Autodesk Fusion 360 part; units mm, degrees
sketch "Sketch1" plane through (0, 0, 0) normal (0, 1, 0) x (1, 0, 0)
  arc A0 (28, 0) -> (-28, 0) centre (0, 0) ccw
  line L0 (-28, 0) -> (-28, -3)
  line L1 (0, -1.75) -> (0, -22.5)
  line L2 (28, 0) -> (28, -3)
  line L3 (-30, 0) -> (-30, -3)
  arc A1 (30, 0) -> (-30, 0) centre (0, 0) ccw
  line L4 (30, 0) -> (30, -3)
  line L5 (-30, -3) -> (-28, -3)
  line L6 (28, -3) -> (30, -3)
  line L7 (-3, 29.8496) -> (-3, 12)
  line L8 (-3, 12) -> (-18, -3)
  line L9 (-18, -3) -> (-28, -3)
  line L10 (18, -3) -> (28, -3)
  line L11 (3, 12) -> (18, -3)
  line L12 (3, 29.8496) -> (3, 12)
  line L13 (-18, -3) -> (18, -3)
  circle A2 centre (0, 4) radius 2
  circle A3 centre (0, 16) radius 2
  dimension "d1" = 28
  dimension "d2" = 3
  dimension "d3" = -2
  dimension "d4" = 135
  dimension "d5" = 6
  dimension "d6" = 15
  dimension "d7" = 7
  dimension "d8" = 12
  dimension "d9" = 4
extrude "Extrude1" add sketch "Sketch1" against normal blind 2
extrude "Extrude2" add sketch "Sketch1" along normal blind 17.5 contours A0 L2 A1 L4 L6 L12 | A0 L0 L3 A1 L5 L7
extrude "Extrude3" add sketch "Sketch1" along normal blind 2 from surface at 17.5 contours A0 L2 L10 L11 L12 | A0 L2 A1 L4 L6 L12 | A0 L0 L7 L8 L9 | A0 L0 L3 A1 L5 L7
fillet "Fillet1" radius 3 2 edges at (3, 0, -28.8442) (-3, 0, -28.8442)
equation "d1 = ( 56 / 2 ) * 1 mm"
Here's how the part is built. I have some questions about the finished solid (model axes, mm). A direction names the side the tool comes from. Give positions to 0.01 mm unless a question says otherwise; leave off trailing zeros. Order: outer loops, then holes, each group sorted by start corner. A loop starts at its lowest first (then second) coordinate and runs counter-clockwise, first axis right, second up. Notation, with made-up numbers: (5, -6.5) - (16, -6.5) arc R26 cw to (16, 19.5) - close; hole circle Ø3 at (38, 33.5). An arc over 180 degrees is marked (long way). Answer as a JSON object with one key per item and string values. Group by question number.
Item 1: Please list where these lines run through material, in increasing order: probe 1 along Z at (x, y) = (0, -1.2); probe 2 along Y at (x, z) = (26, 1.5); probe 3 along X at (y, z) = (-1.15, -16).
Item 2: For P1, Ø10, axis at x = -11.5, y = 6.5, coming from the +Z side; P2, Ø1.5, axis at x = 8, z = -6.5, coming from the +Y side; P3, Ø12, axis at y = 11, z = -19.5, coming from the -X side; P4, Ø1.5, axis at x = 21, y = 2, coming from the +Z side, each with a flat end and sliding along its axis, tell me the tip position at first contact or that it passes through.
Item 3: If we mould it in two halves opening along X, with no side actions, what happens to faces 6 (the flat face through (-17, 19.5, -14)), 7 (the flat face through (10, 18, -5)), 8 (the flat face through (30, 9, 1))? For each: pulls with the +X half, pulls with the -X half, needs draft (parallel to the pull), parting line crosses it, or undercut.
Item 4: If we section it at A-A on y = 18.25: Please give me the cut outline in (x, z).
Item 5: Which directions (+Z, -Z, +X, -X, +Y, -Y) give clear straight access to the entire face, cutting with the end or side of a thin tool? Please do faces 1 (the flat face through (-3, 18, -25)), 2 (the cylindrical face through (0, -1, -2)), 3 (the flat face through (-10, 18, -5)), 4 (the cylindrical face through (19.58, 8.627, -20.015)), 5 (the cylindrical face through (-9.64, 8.9, -28.41)).
Item 6: If we section it at D-D on x = -25.5: Please give me the cut outline in (y, z), and give its area (3 significant figures).
Item 7: If we section it at B-B on z = -16: Please give me the cut outline in (x, y).
Item 8: If we section it at C-C on y = 4.5: Please give me the cut outline in (x, z), and give its area (3 significant figures).
Result set:
{
 "1": {"probe 1": "-30 to -18, -14 to -6, -2 to 3", "probe 2": "-2 to 0, 17.5 to 19.5", "probe 3": "-25.38 to -2, 2 to 25.38"},
 "2": {"P1": "z = -22.62", "P2": "y = 19.5", "P3": "x = -26.79", "P4": "z = -17.63"},
 "3": {"face 6": "needs draft", "face 7": "undercut", "face 8": "pulls with the +X half"},
 "4": {"outline": "(-30, 0) arc R30 ccw to (-3, -29.85) - (-3, -12) - (-18, 3) - (-30, 3) - close; (3, -29.85) arc R30 ccw to (30, 0) - (30, 3) - (18, 3) - (3, -12) - close"},
 "5": {"face 1": "+Z, -Z, +Y", "face 2": "+Y, -Y", "face 3": "+Z, +Y", "face 4": "+Z", "face 5": "-Z, +Y, -Y"},
 "6": {"outline": "(-2, -15.8) - (19.5, -15.8) - (19.5, 3) - (17.5, 3) - (17.5, -11.57) - (0, -11.57) - (0, 3) - (-2, 3) - close", "area": "149 mm²"},
 "7": {"outline": "(-25.38, -2) - (-2, -2) - (-2, 0) - (-22.98, 0) - (-22.98, 17.5) - (-3, 17.5) - (-3, 19.5) - (-25.38, 19.5) - close; (2, -2) - (25.38, -2) - (25.38, 19.5) - (3, 19.5) - (3, 17.5) - (22.98, 17.5) - (22.98, 0) - (2, 0) - close"},
 "8": {"outline": "(-30, 0) arc R30 ccw to (-3, -29.85) - (-3, -27.84) arc R28 cw to (-28, 0) - (-28, 3) - (-30, 3) - close; (3, -29.85) arc R30 ccw to (30, 0) - (30, 3) - (28, 3) - (28, 0) arc R28 cw to (3, -27.84) - close", "area": "182 mm²"}
}
